Read the model definition and answer for the solid it produces. Units are mm, in the model's axes. Face numbers are marked on the shaded views. A direction names the side the tool comes from. Give positions to 0.01 mm unless a question says otherwise; leave off trailing zeros. Order: outer loops, then holes, each group sorted by start corner. A loop starts at its lowest first (then second) coordinate and runs counter-clockwise, first axis right, second up. Notation, with made-up numbers: (-3, 64.5) - (30, 64.5) arc R23 cw to (30, 103.5) - close; hole circle Ø5 at (48, 35.25). An arc over 180 degrees is marked (long way). Answer as CSV lines item,"result". Start each with the question number.
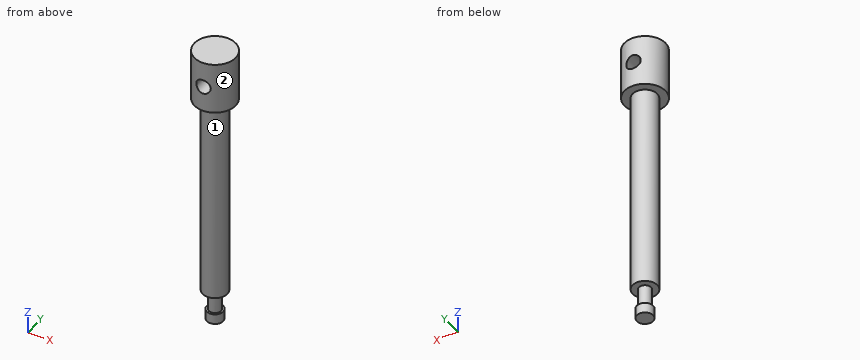
Autodesk Inventor part; units mm, degrees
ref_plane "Work Plane1" through (0, -10, 127.5) normal (0, 1, 0) x (-1, 0, 0)
ref_plane "YZ Plane" through (0, 0, 0) normal (1, 0, 0) x (0, 1, 0)
ref_plane "XY Plane" through (0, 0, 0) normal (0, 0, 1) x (1, 0, 0)
sketch "Sketch1" plane through (0, 0, 0) normal (1, 0, 0) x (0, 1, 0)
  line L0 (0, 140) -> (10, 140)
  line L1 (10, 140) -> (10, 115)
  line L2 (10, 115) -> (6, 115)
  line L3 (6, 115) -> (6, 15)
  line L4 (3, 5) -> (4, 5)
  line L5 (4, 5) -> (4, 0)
  line L6 (4, 0) -> (0, 0)
  line L7 (0, 168) -> (0, -28)
  line L8 (-2, 0) -> (12, 0)
  line L9 (3, 5) -> (3, 15)
  line L10 (3, 15) -> (6, 15)
  line L11 (0, 140) -> (0, 0)
  dimension "d4" = 25
  dimension "d8" = 5
  dimension "d9" = 140
  dimension "d12" = 15
  dimension "d15" = 12
  dimension "d16" = 6
  dimension "d17" = 8
  dimension "d18" = 20
revolve "Revolution1" add sketch "Sketch1" angle 360 about axis through (0, 0, 140) along (0, 0, -1)
ref_plane "Work Plane1" through (0, -10, 127.5) normal (0, 1, 0) x (-1, 0, 0)
sketch "Sketch2" plane through (0, -10, 127.5) normal (0, 1, 0) x (-1, 0, 0)
  line L0 (0, -155.5) -> (0, 40.5)
  line L1 (-10, 12.5) -> (10, 12.5)
  point P0 (0, -127.5)
  point P1 (0, 0)
  dimension "d20" = 12.5
hole "Hole1" at (0, -10, 127.5) direction (0, 1, 0) diameter 7 end through all
thread "Thread1"
properties part number "Spindle"
(1) Straight lines are drawn through the part: line 1 (X direction, y = -0.75, z = 127.5); line 2 (Z direction, x = 0, y = 1); line 3 (Z direction, x = -1.75, y = -3.5). For each, find the intervals that lie inside material, in ascending order. Write a range as [from, to].
(2) Section D-D, the plane z = 127.5 is taken. Write down the section's boundary in (x, y).
(3) Section C-C, the plane z = 108 is taken. Write down the section's boundary in (x, y), and give its area (3 significant figures).
(4) Section A-A, the plane x = 0 is taken. Write down the section's boundary in (y, z), and give its area (3 significant figures).
(5) Which of the six approach directions +Z, -Z, +X, -X, +Y, -Y give full straight-line access (tool end or side, diameter ignored) to the marked faces 1 and 2?
(6) Flat-ended cylindrical pins translate along their axes: pin 1 Ø1 at (y, z) = (3.5, 65) entering from -X; pin 2 Ø1.5 at (x, z) = (-3.5, 88.5) entering from -Y; pin 3 Ø8 at (y, z) = (2, 19) entering from -X. Find the tip coordinate at first contact, or state that the pin passes through.
(7) Section B-B, the plane y = 0 is taken. Write down the section's boundary in (x, z).
Checks:
1,line 1,"x = [-9.97, -3.5], [3.5, 9.97]"
1,line 2,"z = [0, 124], [131, 140]"
1,line 3,"z = [0, 5], [15, 124.47], [130.53, 140]"
2,outline,"(-3.5, -9.37) - (-3.5, 9.37) arc R10 ccw to start; (3.5, -9.37) arc R10 ccw to (3.5, 9.37) - close"
3,outline,"circle Ø12 at (0, 0)"
3,area,"113 mm²"
4,outline,"(-10, 115) - (-6, 115) - (-6, 15) - (-3, 15) - (-3, 5) - (-4, 5) - (-4, 0) - (4, 0) - (4, 5) - (3, 5) - (3, 15) - (6, 15) - (6, 115) - (10, 115) - (10, 124) - (-10, 124) - close; (-10, 131) - (10, 131) - (10, 140) - (-10, 140) - close"
4,area,"1,660 mm²"
5,face 1,"-Z"
5,face 2,"+Z, -Z"
6,pin 1,"stops at x = -5.2"
6,pin 2,"stops at y = -5.33"
6,pin 3,"stops at x = -6"
7,outline,"(-10, 115) - (-6, 115) - (-6, 15) - (-3, 15) - (-3, 5) - (-4, 5) - (-4, 0) - (4, 0) - (4, 5) - (3, 5) - (3, 15) - (6, 15) - (6, 115) - (10, 115) - (10, 140) - (-10, 140) - close; hole circle Ø7 at (0, 127.5)"
